Geometry check sheet. Reference: drawing and pictorial views, mm from the part's lowest x, y, z. A direction names the side the tool comes from. Give positions to 0.01 mm unless a question says otherwise; leave off trailing zeros. Order: outer loops, then holes, each group sorted by start corner. A loop starts at its lowest first (then second) coordinate and runs counter-clockwise, first axis right, second up.
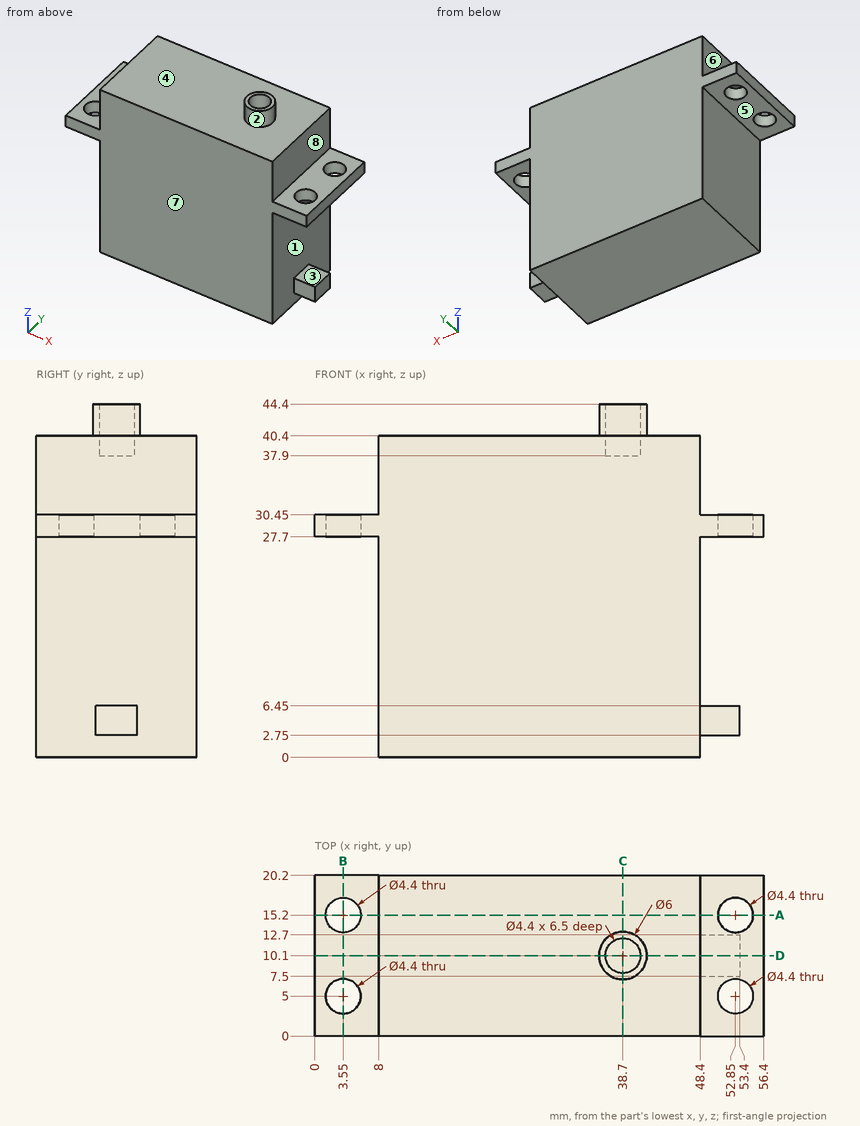
(1) Cross-section at A-A on y = 15.2. Enter the section's corners in (x, z).
Response values:
outline: (0, 27.7) - (1.35, 27.7) - (1.35, 30.45) - (0, 30.45) - close; (5.75, 27.7) - (8, 27.7) - (8, 0) - (48.4, 0) - (48.4, 27.7) - (50.65, 27.7) - (50.65, 30.45) - (48.4, 30.45) - (48.4, 40.4) - (8, 40.4) - (8, 30.45) - (5.75, 30.45) - close; (55.05, 27.7) - (56.4, 27.7) - (56.4, 30.45) - (55.05, 30.45) - close
(2) Cross-section at D-D on y = 10.1. Enter the section's corners in (x, z).
Response values:
outline: (0, 27.7) - (8, 27.7) - (8, 0) - (48.4, 0) - (48.4, 2.75) - (53.4, 2.75) - (53.4, 6.45) - (48.4, 6.45) - (48.4, 27.7) - (56.4, 27.7) - (56.4, 30.45) - (48.4, 30.45) - (48.4, 40.4) - (41.7, 40.4) - (41.7, 44.4) - (40.9, 44.4) - (40.9, 37.9) - (36.5, 37.9) - (36.5, 44.4) - (35.7, 44.4) - (35.7, 40.4) - (8, 40.4) - (8, 30.45) - (0, 30.45) - close
(3) Set-up check for the marked faces 5, 6, 7 and 8: record each of +Z, -Z, +X, -X, +Y, -Y from which the full face is reachable in a straight line by a thin tool's end or side.
Response values:
face 5: -Z, -X, +Y, -Y
face 6: +Z, -X, +Y, -Y
face 7: +Z, -Z, +X, -X, -Y
face 8: +Z, +X, +Y, -Y
(4) Material ranges on L1, parallel to X at y = 5, z = 29.4; L2, parallel to Y at x = 52.85, z = 29.2; L3, parallel to X at y = 10.1, z = 41.5, recorded low to high.
Response values:
L1: x = 0 to 1.35, 5.75 to 50.65, 55.05 to 56.4
L2: y = 0 to 2.8, 7.2 to 13, 17.4 to 20.2
L3: x = 35.7 to 36.5, 40.9 to 41.7
(5) Cross-section at C-C on x = 38.7. Enter the section's corners in (y, z).
Response values:
outline: (0, 0) - (20.2, 0) - (20.2, 40.4) - (13.1, 40.4) - (13.1, 44.4) - (12.3, 44.4) - (12.3, 37.9) - (7.9, 37.9) - (7.9, 44.4) - (7.1, 44.4) - (7.1, 40.4) - (0, 40.4) - close
(6) Gauge pin test, flat ends, axial feed: pin 1 Ø11 at (y, z) = (6.5, 38) entering from -X; pin 2 Ø4 at (x, y) = (51.5, 8.5) entering from +Z; pin 3 Ø5.5 at (x, y) = (52.85, 15.2) entering from -Z. Record the tip position at first contact, or that the pin passes through.
Response values:
pin 1: stops at x = 8
pin 2: stops at z = 30.45
pin 3: stops at z = 2.75
(7) Cross-section at B-B on x = 3.55. Enter the section's corners in (y, z).
Response values:
outline: (0, 27.7) - (2.8, 27.7) - (2.8, 30.45) - (0, 30.45) - close; (7.2, 27.7) - (13, 27.7) - (13, 30.45) - (7.2, 30.45) - close; (17.4, 27.7) - (20.2, 27.7) - (20.2, 30.45) - (17.4, 30.45) - close
(8) Release check for a two-part mould opening along Z. For the marked faces 1, 2, 3 and 4 record: released by +Z, released by -Z, zero draft, split by the parting line, or undercut.
Response values:
face 1: undercut
face 2: zero draft
face 3: undercut
face 4: released by +Z
